Source: CAD feature listing. Evaluate the final solid. Frame: model axes, mm. A direction names the side the tool comes from. Round coordinates to 2 decimals unless told otherwise and drop trailing zeros. Loops run counter-clockwise (first coordinate to the right, second up) from the corner with the lowest first, then second, coordinate; pieces in that order, holes last.
(1) Material intervals for probe 1 along X at (y, z) = (1.5, 2); probe 2 along Z at (x, y) = (21, 0.25); probe 3 along Z at (x, y) = (13, 0.5), sorted ascending.
(2) Section D-D, the plane y = -2.5. Return the cut outline in (x, z), plus the area to 3 significant figures.
(3) First-contact query: pin 1 Ø3 at (x, z) = (9.5, -1.5) entering from +Y; pin 2 Ø2 at (x, y) = (-4.5, 0) entering from -Z; pin 3 Ø4 at (x, z) = (2, 0.5) entering from -Y. Flat tips, straight axial feed; report the tip coordinate or a pass-through.
(4) Section C-C, the plane x = 11. Return the cut outline in (y, z) (1 decimal), plus the area to 3 significant figures.
(5) Set-up query: faces 1 (the flat face through (26.746, 0, 0)), 2 (the flat face through (16.154, 0, -2)). Return all of +Z, -Z, +X, -X, +Y, -Y with unobstructed straight access to the full face (end or side cutting, diameter ignored); none if empty.
(6) Section A-A, the plane y = 0. Return the cut outline in (x, z), plus the area to 3 significant figures.
Autodesk Inventor part; units mm, degrees
ref_plane "dia1_XY" through (0, 1.5875, 0) normal (1, 0, 0) x (0, 0, -1)
ref_plane "dia1_YZ" through (0, 1.5875, 0) normal (0, 0, -1) x (0, 1, 0)
ref_plane "dia1_ZX" through (0, 1.5875, 0) normal (0, 1, 0) x (1, 0, 0)
sketch "Sketch_1" plane through (0, 0, 0) normal (0, 0, 1) x (1, 0, 0)
  line L0 (26.7462, 0) -> (0, 0)
  line L1 (0, 0) -> (0, 1.5875)
  line L2 (0, 1.5875) -> (16.1544, 1.5875)
  line L3 (16.1544, 1.5875) -> (16.1544, 4.0323)
  line L4 (16.1544, 4.0323) -> (26.7462, 4.0323)
  line L5 (26.7462, 4.0323) -> (26.7462, 0)
  line L6 (26.7462, 0) -> (0, 0)
revolve "Revolution1" add sketch "Sketch_1" angle 360 about axis through (26.7462, 0, 0) along (1, 0, 0)
sketch "Sketch_2" plane through (0, 0, 0) normal (0, 0, 1) x (1, 0, 0)
  line L0 (0, 0) -> (-9.652, 0)
  line L1 (-9.652, 0) -> (-9.652, 1.209)
  line L2 (-9.652, 1.209) -> (-9.2735, 1.5875)
  line L3 (-9.2735, 1.5875) -> (0, 1.5875)
  line L4 (0, 1.5875) -> (0, 0)
  line L5 (0, 0) -> (-9.652, 0)
revolve "Revolution2" add sketch "Sketch_2" angle 360 about axis through (0, 0, 0) along (1, 0, 0)
thread "Thread1"
sketch "Sketch_30" plane through (0, 0, 0) normal (0, 0, 1) x (1, 0, 0)
  line L0 (0, 0) -> (-0.254, 0)
  line L1 (-0.254, 1.3335) -> (0, 1.3335)
  line L2 (0, 1.3335) -> (0, 1.8415)
  line L3 (0, 1.8415) -> (-0.254, 1.8415)
  line L4 (-0.254, 1.8415) -> (-0.254, 1.3335)
revolve "Revolution3" cut sketch "Sketch_30" angle 360 about axis through (0, 0, 0) along (1, 0, 0)
ref_plane "dia1_XY" through (0, 1.5875, 0) normal (1, 0, 0) x (0, 0, -1)
ref_plane "dia1_YZ" through (0, 1.5875, 0) normal (0, 0, -1) x (0, 1, 0)
ref_plane "dia1_ZX" through (0, 1.5875, 0) normal (0, 1, 0) x (1, 0, 0)
ref_plane "dia12_XY" through (0, 0, 4.5593) normal (1, 0, 0) x (0, 0, -1)
ref_plane "dia12_YZ" through (0, 0, 4.5593) normal (0, 0, -1) x (0, 1, 0)
ref_plane "dia12_ZX" through (0, 0, 4.5593) normal (0, 1, 0) x (1, 0, 0)
ref_plane "dia2_XY" through (0, -1.5875, 0) normal (1, 0, 0) x (0, 0, -1)
ref_plane "dia2_YZ" through (0, -1.5875, 0) normal (0, 0, -1) x (0, 1, 0)
ref_plane "dia2_ZX" through (0, -1.5875, 0) normal (0, 1, 0) x (1, 0, 0)
ref_plane "dia22_XY" through (0, 0, -4.5593) normal (1, 0, 0) x (0, 0, -1)
ref_plane "dia22_YZ" through (0, 0, -4.5593) normal (0, 0, -1) x (0, 1, 0)
ref_plane "dia22_ZX" through (0, 0, -4.5593) normal (0, 1, 0) x (1, 0, 0)
ref_plane "rl1_XY" through (-9.652, 0, 0) normal (1, 0, 0) x (0, 0, -1)
ref_plane "rl1_YZ" through (-9.652, 0, 0) normal (0, 0, -1) x (0, 1, 0)
ref_plane "rl1_ZX" through (-9.652, 0, 0) normal (0, 1, 0) x (1, 0, 0)
ref_plane "rl2_XY" through (0, 0, 0) normal (1, 0, 0) x (0, 0, -1)
ref_plane "rl2_YZ" through (0, 0, 0) normal (0, 0, -1) x (0, 1, 0)
ref_plane "rl2_ZX" through (0, 0, 0) normal (0, 1, 0) x (1, 0, 0)
ref_plane "rod_cp_XY" through (0, 0, 0) normal (1, 0, 0) x (0, 0, -1)
ref_plane "rod_cp_YZ" through (0, 0, 0) normal (0, 0, -1) x (0, 1, 0)
ref_plane "rod_cp_ZX" through (0, 0, 0) normal (0, 1, 0) x (1, 0, 0)
ref_plane "thd1_XY" through (-9.652, 1.5875, 0) normal (1, 0, 0) x (0, 0, -1)
ref_plane "thd1_YZ" through (-9.652, 1.5875, 0) normal (0, 0, -1) x (0, 1, 0)
ref_plane "thd1_ZX" through (-9.652, 1.5875, 0) normal (0, 1, 0) x (1, 0, 0)
ref_plane "thd2_XY" through (-9.652, -1.5875, 0) normal (1, 0, 0) x (0, 0, -1)
ref_plane "thd2_YZ" through (-9.652, -1.5875, 0) normal (0, 0, -1) x (0, 1, 0)
ref_plane "thd2_ZX" through (-9.652, -1.5875, 0) normal (0, 1, 0) x (1, 0, 0)
ref_plane "to_rod_clevis_XY" through (-9.652, 0, 0) normal (1, 0, 0) x (0, 0, -1)
ref_plane "to_rod_clevis_YZ" through (-9.652, 0, 0) normal (0, 0, -1) x (0, 1, 0)
ref_plane "to_rod_clevis_ZX" through (-9.652, 0, 0) normal (0, 1, 0) x (1, 0, 0)
properties part number "0070.0110000_rod"
Output values:
1. probe 1: x = 16.15 to 26.75
1. probe 2: z = -4.02 to 4.02
1. probe 3: z = -1.51 to 1.51
2. outline: (16.15, -3.16) - (26.75, -3.16) - (26.75, 3.16) - (16.15, 3.16) - close
2. area: 67.0 mm2
3. pin 1: stops at y = 1.59
3. pin 2: stops at z = -1.59
3. pin 3: stops at y = -1.59
4. outline: circle Ø3.2 at (0, 0)
4. area: 7.92 mm2
5. face 1: +Z, -Z, +X, +Y, -Y
5. face 2: -X
6. outline: (-9.65, -1.21) - (-9.27, -1.59) - (-0.25, -1.59) - (-0.25, -1.33) - (0, -1.33) - (0, -1.59) - (16.15, -1.59) - (16.15, -4.03) - (26.75, -4.03) - (26.75, 4.03) - (16.15, 4.03) - (16.15, 1.59) - (0, 1.59) - (0, 1.33) - (-0.25, 1.33) - (-0.25, 1.59) - (-9.27, 1.59) - (-9.65, 1.21) - close
6. area: 167 mm2
